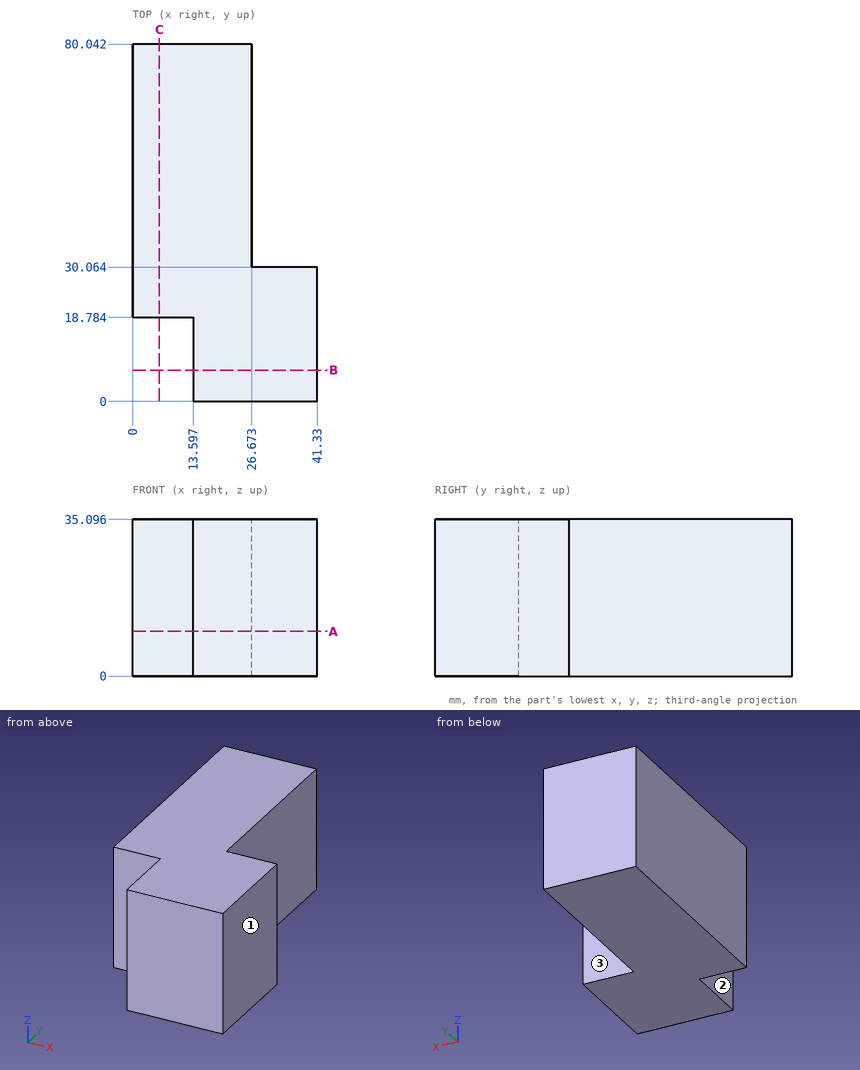
Drawing for the job (mm, zero at the part's lowest x, y, z). A direction names the side the tool comes from. Round coordinates to 2 decimals unless told otherwise and drop trailing zeros. Order: outer loops, then holes, each group sorted by start corner. A loop starts at its lowest first (then second) coordinate and runs counter-clockwise, first axis right, second up. Notation, with made-up numbers: M -14,-12 L 41,-12 A13 ccw 41,-6 Z; hole C 57,-18 d6. An arc over 180 degrees is marked long. Use one line per item in the form item = value.
Q1. Saw through at B-B on y = 7. Give the cut face in (x, z), then the cut area to 3 significant figures.
Recorded:
outline = M 13.6,0 L 41.33,0 L 41.33,35.1 L 13.6,35.1 Z
area = 973 mm^2
Q2. Probe L1, parallel to X at y = 71, z = 1; L2, parallel to Y at x = 39, z = 26; L3, parallel to Y at x = 7, z = 4.5. List the from-to ranges inside material, lowest first.
Recorded:
L1 = 0 to 26.67
L2 = 0 to 30.06
L3 = 18.78 to 80.04
Q3. Flat gauge pins, fed straight in: P1, Ø10, axis at y = 38, z = 10, coming from the +X side; P2, Ø20.5, axis at y = 5, z = 24.5, coming from the -X side; P3, Ø12, axis at x = 36, y = 26, coming from the -Z side; P4, Ø3, axis at x = 31.5, z = 7.5, coming from the +Y side. Where does each tip first touch, or does it go through?
Recorded:
P1 = 26.67
P2 = 13.6
P3 = 0
P4 = 30.06
Q4. Which spindle directions (+Z, -Z, +X, -X, +Y, -Y) get a long thin tool onto all of the face, cutting with end or side? Do the marked faces 1, 2 and 3. Say none if no direction does.
Recorded:
face_1 = +Z, -Z, +X, +Y, -Y
face_2 = +Z, -Z, -X, -Y
face_3 = +Z, -Z, +X, +Y
Q5. Saw through at C-C on x = 6. Give the cut face in (y, z), then the cut area to 3 significant figures.
Recorded:
outline = M 18.78,0 L 80.04,0 L 80.04,35.1 L 18.78,35.1 Z
area = 2,150 mm^2
Q6. Saw through at A-A on z = 10. Give the cut face in (x, y), then the cut area to 3 significant figures.
Recorded:
outline = M 0,18.78 L 13.6,18.78 L 13.6,0 L 41.33,0 L 41.33,30.06 L 26.67,30.06 L 26.67,80.04 L 0,80.04 Z
area = 2,320 mm^2
